from build123d import *

# Parameters (mm, degrees)
ESQUISSE1_W             = 3
ESQUISSE1_H             = 1
LANGUETTE_PLI_E_DEPTH   = 2
LANGUETTE_DEPTH         = 2
NBR_DE_LANGUETTES_COUNT = 12
NBR_DE_LANGUETTES_ANGLE = 304.615384615


with BuildPart() as part:
    # Esquisse1 → Base (revolve)
    with BuildSketch(Plane.XY, mode=Mode.PRIVATE) as base_sk:
        with Locations((11.5, 0.5)):
            Rectangle(ESQUISSE1_W, ESQUISSE1_H)
    revolve(base_sk.sketch.rotate(Axis((0, 0, 0), (0, 1, 0)), 90), axis=Axis((0, 0, 0), (0, 1, 0)))

    # Esquisse3 → Languette pliée (add, symmetric)
    with BuildSketch(Plane(origin=(0, 0, 0), x_dir=(0, 0, -1), z_dir=(1, 0, 0))):
        with BuildLine():
            Line((13.5, 5), (13.5, 1.5))
            ThreePointArc((13.5, 1.5), (13.353553391, 1.146446609), (13, 1))
            Line((13, 1), (10, 1))
            Line((10, 1), (8.5, 1))
            Line((8.5, 1), (8.5, 0))
            Line((8.5, 0), (10, 0))
            Line((10, 0), (13, 0))
            ThreePointArc((13, 0), (14.060660172, 0.439339828), (14.5, 1.5))
            Line((14.5, 1.5), (14.5, 5))
            Line((14.5, 5), (13.5, 5))
        make_face()
    extrude(amount=LANGUETTE_PLI_E_DEPTH, both=True)

    # Esquisse2 → Languette (add, symmetric)
    with BuildSketch(Plane(origin=(0, 0, 0), x_dir=(-0.46472317204377556, 0, 0.8854560256532064), z_dir=(-0.8854560256532064, 0, -0.46472317204377556))):
        with BuildLine():
            Line((-10, 1), (-12.577381738, 1))
            ThreePointArc((-12.577381738, 1), (-12.685601545, 1.011851996), (-12.788690869, 1.046846106))
            Line((-12.788690869, 1.046846106), (-17.788690869, 3.378384397))
            Line((-17.788690869, 3.378384397), (-18.211309131, 2.47207661))
            Line((-18.211309131, 2.47207661), (-13.211309131, 0.140538319))
            ThreePointArc((-13.211309131, 0.140538319), (-12.902041159, 0.035555989), (-12.577381738, 0))
            Line((-12.577381738, 0), (-10, 0))
            Line((-10, 0), (-10, 1))
        make_face()
    languette = extrude(amount=LANGUETTE_DEPTH, both=True)

    # Nbr de languettes: Languette ×12 about axis
    nbr_de_languettes_axis = Axis((0, 0, 0), (0, -1, 0))
    for i in range(1, NBR_DE_LANGUETTES_COUNT):
        add(languette.rotate(nbr_de_languettes_axis, i * NBR_DE_LANGUETTES_ANGLE / (NBR_DE_LANGUETTES_COUNT - 1)))


solid = part.part
Can you work these out from the model? Positions are in its coordinate system, mm. A direction names the side the tool comes from. Give positions to 0.01 mm unless a question says otherwise; leave off trailing zeros. Order: outer loops, then holes, each group sorted by start corner. A loop starts at its lowest first (then second) coordinate and runs counter-clockwise, first axis right, second up. Notation, with made-up numbers: M 41,21.5 L 57,21.5 A31 ccw 57,48.5 Z; hole C 41,-18 d9. An arc over 180 degrees is marked long. One line per question, with ' | ' between items.
Item 1: Suppose I cut it at C-C, the plane z = 14. Write out the boundary of the cut face in (x, y).
Answer block:
outline: M -11.66,2.47 L -9.73,1.88 L -9.73,2.98 L -11.02,3.38 Z; M -5.51,0.93 L -1.39,0.47 L -1.39,1.58 L -5.51,2.04 Z; M 1.39,0.47 L 5.51,0.93 L 5.51,2.04 L 1.39,1.58 Z; M 9.73,1.88 L 11.66,2.47 L 11.02,3.38 L 9.73,2.98 Z
Item 2: Please list where these lines run through material, in increasing order: L1, parallel to Z at x = 0, y = 0.4; L2, parallel to X at y = 0.65, z = 0; L3, parallel to X at y = 0.55, z = 0.
Answer block:
L1: z = -14.02 to -8.5, 10 to 13 | L2: x = -14.41 to -10, 10 to 14.41 | L3: x = -14.19 to -10, 10 to 14.19
Item 3: We'd pull the mould along Z, two halves only. Please class faces 1 (the face through (-15.115, 1.833, 3.594)), 2 (the face through (-12.97, 1.32, -8.92)), 3 (the face through (-1.745, 1.833, 15.438)): released by +Z, released by -Z, zero draft, split by the parting line, or undercut.
Answer block:
face 1: undercut | face 2: released by -Z | face 3: released by +Z
Item 4: Suppose I cut it at D-D, the plane y = 4.2. Write out the boundary of the cut face in (x, z), then the cut area to 3 significant figures.
Answer block:
outline: M -2,-14.5 L 2,-14.5 L 2,-13.5 L -2,-13.5 Z | area: 4.00 mm2
Item 5: I'm going to push flat-ended pins straight in: pin 1 Ø0.8 at (x, y) = (0.5, 0.5) entering from +Z; pin 2 Ø1 at (x, z) = (0.5, 11) entering from +Y; pin 3 Ø1 at (x, y) = (0, 3.5) entering from -Z. Where does each tip first touch, or does it pass through?
Answer block:
pin 1: stops at z = 13 | pin 2: stops at y = 1 | pin 3: stops at z = -14.5
Item 6: For faces 4 (the face through (-7.3, 1.3, -13.9)), 5 (the face through (11.714, 1.833, 10.206)), 6 (the face through (-14.253, 2.196, 5.435)), which set-ups out of +Z, -Z, +X, -X, +Y, -Y let a thin tool reach every point of the face, with its end or its side?
Answer block:
face 4: -Z, -X, -Y | face 5: +X, +Y, -Y | face 6: +Y
Item 7: Suppose I cut it at A-A, the plane x = 0. Write out the boundary of the cut face in (y, z).
Answer block:
outline: M 0,-13 A1.5 ccw 1.5,-14.5 L 5,-14.5 L 5,-13.5 L 1.5,-13.5 A0.5 cw 1,-13 L 1,-8.5 L 0,-8.5 Z; M 0,10 L 1,10 L 1,13 L 0,13 Z
Item 8: Suppose I cut it at B-B, the plane x = -15. Write out the boundary of the cut face in (y, z).
Answer block:
outline: M 0.91,0.19 L 1.14,-3.84 L 2.24,-3.84 L 2.02,0.19 Z; M 1.11,3.55 L 2.21,3.55 L 2.92,7.83 L 1.81,7.83 Z; M 1.84,-7.92 L 2.47,-10.33 L 3.38,-9.58 L 2.94,-7.92 Z
